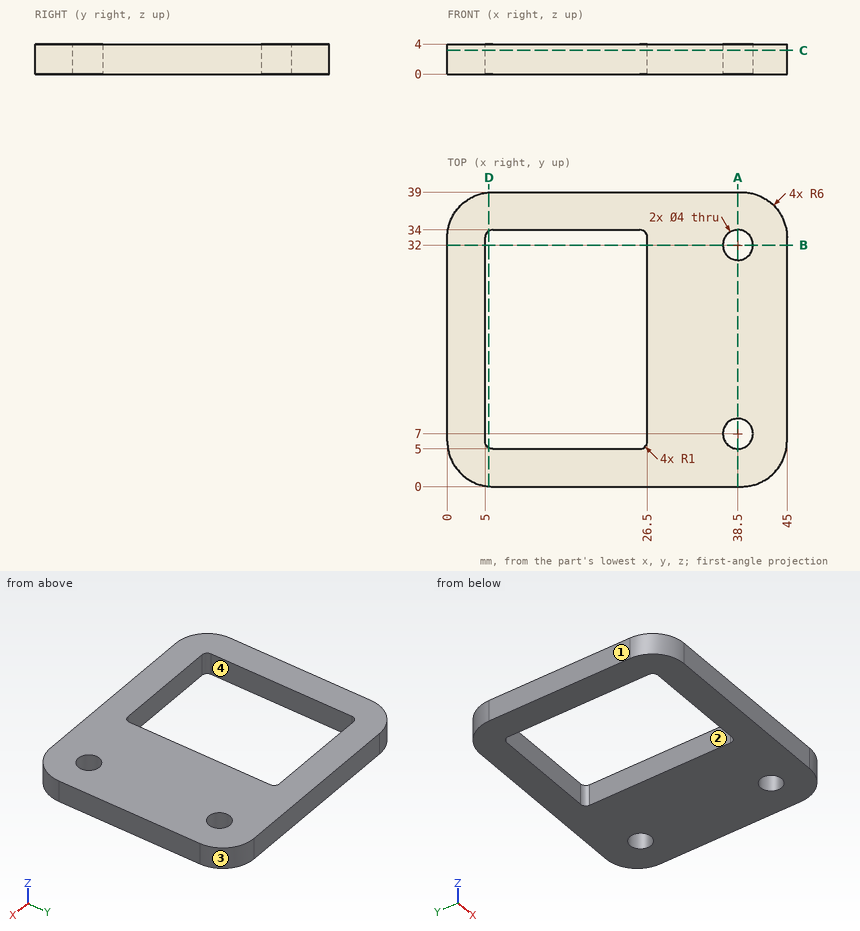
Part print with two shaded views. Sizes in mm from the minimum x, y, z corner. Round coordinates to 2 decimals unless told otherwise and drop trailing zeros. Order: outer loops, then holes, each group sorted by start corner. A loop starts at its lowest first (then second) coordinate and runs counter-clockwise, first axis right, second up. Notation, with made-up numbers: M 69.25,58 L 103.25,58 A20 ccw 103.25,77 Z; hole C 65.5,16 d10. An arc over 180 degrees is marked long. Use CSV: the item, a comma, the result in double quotes. Start each with the question number.
(1) Mould opens along Y. For the marked faces 1, 2, 3 and 4 say: +Y half, -Y half, draft (parallel to the pull), parting line (faces both ways), or undercut.
(2) Cut at D-D on x = 5.5. List the corners of the cut face in (y, z), then the cut area to 3 significant figures.
(3) Flat gauge pin, fed straight in: P1, Ø1, axis at y = 4, z = 1.5, coming from the -X side. Where does the tip first touch, or does it go through?
(4) Cut at C-C on z = 3.15. List the corners of the cut face in (x, y).
(5) Drill centre lines: probe 1 along Y at (x, z) = (38.5, 2.8); probe 2 along Y at (x, z) = (10.5, 2.8); probe 3 along X at (y, z) = (13.5, 2.95). Where is each one in solid material? Low to high.
(6) Cut at B-B on y = 32. List the corners of the cut face in (x, z), then the cut area to 3 significant figures.
(7) Cut at A-A on x = 38.5. List the corners of the cut face in (y, z), then the cut area to 3 significant figures.
Findings:
1,face 1,"draft"
1,face 2,"undercut"
1,face 3,"+Y half"
1,face 4,"undercut"
2,outline,"M 0.02,0 L 5.13,0 L 5.13,4 L 0.02,4 Z; M 33.87,0 L 38.98,0 L 38.98,4 L 33.87,4 Z"
2,area,"40.9 mm^2"
3,P1,"stops at x = 0.19"
4,outline,"M 0,6 A6 ccw 6,0 L 39,0 A6 ccw 45,6 L 45,33 A6 ccw 39,39 L 6,39 A6 ccw 0,33 Z; hole M 5,6 A1 ccw 6,5 L 25.5,5 A1 ccw 26.5,6 L 26.5,33 A1 ccw 25.5,34 L 6,34 A1 ccw 5,33 Z; hole C 38.5,7 d4; hole C 38.5,32 d4"
5,probe 1,"y = 0 to 5, 9 to 30, 34 to 39"
5,probe 2,"y = 0 to 5, 34 to 39"
5,probe 3,"x = 0 to 5, 26.5 to 45"
6,outline,"M 0,0 L 5,0 L 5,4 L 0,4 Z; M 26.5,0 L 36.5,0 L 36.5,4 L 26.5,4 Z; M 40.5,0 L 45,0 L 45,4 L 40.5,4 Z"
6,area,"78.0 mm^2"
7,outline,"M 0,0 L 5,0 L 5,4 L 0,4 Z; M 9,0 L 30,0 L 30,4 L 9,4 Z; M 34,0 L 39,0 L 39,4 L 34,4 Z"
7,area,"124 mm^2"
